Verification items for the finished model (mm, model axes). Face numbers are marked on the shaded views. A direction names the side the tool comes from. Give positions to 0.01 mm unless a question says otherwise; leave off trailing zeros. Loops run counter-clockwise (first coordinate to the right, second up) from the corner with the lowest first, then second, coordinate; pieces in that order, holes last. Notation, with made-up numbers: (-39.5, -19) -> (-5.5, -19) arc R27 ccw to (-5.5, 17) -> close; hole circle Ø1 at (-3.5, 40). An arc over 180 degrees is marked (long way). Answer in a Markdown table with one row per item. Add a question column.
Q1. Section check C-C on x = -12. Give the number of separate pieces and of enclosed holes in the cut face, and give its area (3 significant figures).
Q2. Section check B-B on y = 19. Enter the section's corners in (x, z), and give its area (3 significant figures).
Q3. Set-up check for the marked faces 5 and 6: record each of +Z, -Z, +X, -X, +Y, -Y from which the full face is reachable in a straight line by a thin tool's end or side.
Q4. Section check A-A on x = 0. Enter the section's corners in (y, z), and give its area (3 significant figures).
Q5. Release check for a two-part mould opening along Z. For the marked faces 1, 2, 3 and 4 record: pulls with the +Z half, pulls with the -Z half, needs draft (parallel to the pull), parting line crosses it, or undercut.
Q6. Gauge pin test, flat ends, axial feed: P1, Ø6.5, axis at x = 13.44, z = 13.44, coming from the +Y side; P2, Ø8, axis at x = 13.5, y = 3, coming from the +Z side; P3, Ø10, axis at x = 3.5, z = 5, coming from the +Y side; P4, Ø5, axis at x = 5.5, y = 9, coming from the +Z side. Record the tip position at first contact, or that the pin passes through.
Q7. Material ranges on probe 1 along Z at (x, y) = (0, -3.5); probe 2 along Y at (x, z) = (8, 19.5); probe 3 along X at (y, z) = (-2, -17), recorded low to high.
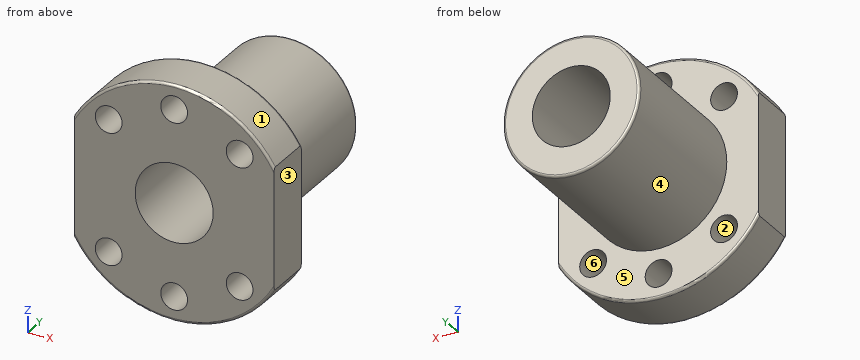
```python
from build123d import *

# Parameters (mm, degrees)
F1_DEPTH = 10
F2_R     = 2.75
F3_DEPTH = 10.001
F4_R     = 14
F5_DEPTH = 32
F6_R     = 8
F7_DEPTH = 42.001
F8_R     = 0.5


with BuildPart() as f1:
    # F0 (on Front) → F1 (new body)
    with BuildSketch(Plane.XZ):
        with BuildLine():
            Line((-20.5, 12.479984), (-20.5, -12.479984))
            ThreePointArc((-20.5, -12.479984), (0, -24), (20.5, -12.479984))
            Line((20.5, -12.479984), (20.5, 12.479984))
            ThreePointArc((20.5, 12.479984), (0, 24), (-20.5, 12.479984))
        make_face()
    extrude(amount=F1_DEPTH)

    # F2 (on face) → F3 (cut, through all)
    with BuildSketch(Plane.XZ.offset(10)):
        with Locations((0, 19)):
            Circle(F2_R)
        with Locations((-13.435029, 13.435029)):
            Circle(F2_R)
        with Locations((13.435029, -13.435029)):
            Circle(F2_R)
        with Locations((13.435029, 13.435029)):
            Circle(F2_R)
        with Locations((-13.435029, -13.435029)):
            Circle(F2_R)
        with Locations((0, -19)):
            Circle(F2_R)
    extrude(amount=-F3_DEPTH, mode=Mode.SUBTRACT)

    # F4 (on face) → F5 (join)
    with BuildSketch(Plane(origin=(0, 0, 0), x_dir=(-1, 0, 0), z_dir=(0, 1, 0))):
        Circle(F4_R)
    extrude(amount=F5_DEPTH)

    # F6 (on face) → F7 (cut, through all)
    with BuildSketch(Plane.XZ.offset(10)):
        Circle(F6_R)
    extrude(amount=-F7_DEPTH, mode=Mode.SUBTRACT)

    # F8
    f8_edges = [f1.edges().sort_by_distance(p)[0] for p in [
        (14, 32, 0),
        (0, 0, 24),
        (0, 0, -24),
        (0, -10, -24),
        (0, -10, 24),
    ]]
    fillet(f8_edges, radius=F8_R)


solid = f1.part
```
Taken from the geometry:
| question | item | result |
|---|---|---|
| 1 | separate pieces | 3 |
| 1 | enclosed holes | 0 |
| 1 | area | 783 mm² |
| 2 | outline | circle Ø28 at (0, 0); hole circle Ø16 at (0, 0) |
| 2 | area | 415 mm² |
| 3 | face 5 | +Y |
| 3 | face 6 | +Y, -Y |
| 4 | outline | (-10, -23.5) arc R0.5 ccw to (-9.5, -24) -> (-0.5, -24) arc R0.5 ccw to (0, -23.5) -> (0, -21.75) -> (-10, -21.75) -> close; (-10, -16.25) -> (0, -16.25) -> (0, -14) -> (31.5, -14) arc R0.5 ccw to (32, -13.5) -> (32, -8) -> (-10, -8) -> close; (-10, 8) -> (32, 8) -> (32, 13.5) arc R0.5 ccw to (31.5, 14) -> (0, 14) -> (0, 16.25) -> (-10, 16.25) -> close; (-10, 21.75) -> (0, 21.75) -> (0, 23.5) arc R0.5 ccw to (-0.5, 24) -> (-9.5, 24) arc R0.5 ccw to (-10, 23.5) -> close |
| 4 | area | 594 mm² |
| 5 | face 1 | pulls with the +Z half |
| 5 | face 2 | undercut |
| 5 | face 3 | needs draft |
| 5 | face 4 | parting line crosses it |
| 6 | P1 | stops at y = 0 |
| 6 | P2 | stops at z = 21.17 |
| 6 | P3 | stops at y = 32 |
| 6 | P4 | stops at z = 13.67 |
| 7 | probe 1 | z = -24 to -21.75, -16.25 to -8, 8 to 16.25, 21.75 to 24 |
| 7 | probe 2 | y = -10 to 0 |
| 7 | probe 3 | x = -16.94 to -1.89, 1.89 to 16.94 |
